from build123d import *

# Parameters (mm, degrees)
F0_R     = 31.4391719437
F1_DEPTH = 5.08
F2_T     = -2.54
F4_DEPTH = 2.54


# Not quite as in the source:
# - a feature names something its author has since deleted; it is built from what else it names


with BuildPart() as f1:
    # F0 (on Top) → F1 (new body)
    with BuildSketch(Plane.XY):
        Circle(F0_R)
    extrude(amount=F1_DEPTH)

    # F2
    f2_openings = [f1.faces().sort_by_distance(p)[0] for p in [
        (0, 0, 5.08),
    ]]
    offset(amount=F2_T, openings=f2_openings)

    # F3 (on face) → F4 (join)
    with BuildSketch(Plane.XY.offset(2.54)):
        with BuildLine():
            Line((-13.4078683332, 0), (-28.8991719437, 0))
            ThreePointArc((-28.8991719437, 0), (-24.7248703878, -14.9613810638), (-13.4078683332, -25.6006094808))
            Line((-13.4078683332, -25.6006094808), (-13.4078683332, 0))
        make_face()
        with BuildLine():
            ThreePointArc((28.8991719437, 0), (24.9790772251, 14.5329914336), (14.2822936177, 25.1232606969))
            Line((14.2822936177, 25.1232606969), (14.2822936177, 0))
            Line((14.2822936177, 0), (28.8991719437, 0))
        make_face()
    extrude(amount=F4_DEPTH)


solid = f1.part
Work out the finished part from the listing and answer in its coordinate system (mm). A direction names the side the tool comes from. Coordinates: 2 decimals unless noted, no trailing zeros. Write each loop counter-clockwise with the first axis right and the second up, starting at its lowest first coordinate (ties: lowest second). Pieces come first, ordered by that corner, then holes. Notation, with made-up numbers: M 43.5,85 L 73.5,85 A21 cw 73.5,90 Z; hole C 61.5,41.25 d4. An arc over 180 degrees is marked long. Write item = value, one per line.
1. Determine the mould class of faces 3 (the face through (14.282, 13, 4)), 4 (the face through (-14, -5, 5.08)), 5 (the face through (30, 9.4, 2.5)) for opening direction Y: released by +Y, released by -Y, zero draft, split by the parting line, or undercut.
Solution:
face_3 = undercut
face_4 = zero draft
face_5 = split by the parting line
2. The part is cut by section C-C (z = 1). Determine the outline of the cut face in (x, y), then the cut area to 3 significant figures.
Solution:
outline = C 0,0 d62.88
area = 3,110 mm2
3. The part is cut by section A-A (x = 0). Determine the outline of the cut face in (y, z), then the cut area to 3 significant figures.
Solution:
outline = M -31.44,0 L 31.44,0 L 31.44,5.08 L 28.9,5.08 L 28.9,2.54 L -28.9,2.54 L -28.9,5.08 L -31.44,5.08 Z
area = 173 mm2
4. Straight lines are drawn through the part: line 1 (Y direction, x = 0, z = 3.8); line 2 (Z direction, x = -27, y = 2); line 3 (Y direction, x = -25, z = 3.2). For each, find the intervals that lie inside material, in ascending order. Write a range as from..to.
Solution:
line_1 = -31.44..-28.9, 28.9..31.44
line_2 = 0..2.54
line_3 = -19.06..0, 14.5..19.06
5. The part is cut by section B-B (y = -10). Determine the outline of the cut face in (x, z), then the cut area to 3 significant figures.
Solution:
outline = M -29.81,0 L 29.81,0 L 29.81,5.08 L 27.11,5.08 L 27.11,2.54 L -13.41,2.54 L -13.41,5.08 L -29.81,5.08 Z
area = 200 mm2
6. For faces 1 (the face through (-14.166, 25.189, 3.792)), 2 (the face through (0, 0, 0)), determine the directions among +Z, -Z, +X, -X, +Y, -Y from which every point of the face is accessible in a straight line to the end or side of a thin tool.
Solution:
face_1 = +Z
face_2 = -Z, +X, -X, +Y, -Y
7. Flat-ended cylindrical pins translate along their axes: pin 1 (2 mm diameter, centred on x = 25, z = 4, fed in from -Y); pin 2 (1.5 mm diameter, centred on y = 21, z = 4, fed in from -X); pin 3 (1.3 mm diameter, centred on y = -13, z = 3.5, fed in from +X); pin 4 (1.5 mm diameter, centred on x = 7, y = -20, fed in from -Z). Find the tip coordinate at first contact, or state that the pin passes through.
Solution:
pin_1 = -20.31
pin_2 = -24.05
pin_3 = 28.91
pin_4 = 0
